Source: three-view drawing plus pictorial views. Frame: mm from the lowest corner of the part. Round coordinates to 2 decimals unless told otherwise and drop trailing zeros. Loops run counter-clockwise (first coordinate to the right, second up) from the corner with the lowest first, then second, coordinate; pieces in that order, holes last. Notation, with made-up numbers: M -18.75,27.5 L 13.25,27.5 A27 cw 13.25,49.5 Z; hole C -37,56.25 d5. An arc over 180 degrees is marked long. Answer as a JSON object with one key per item and string values.
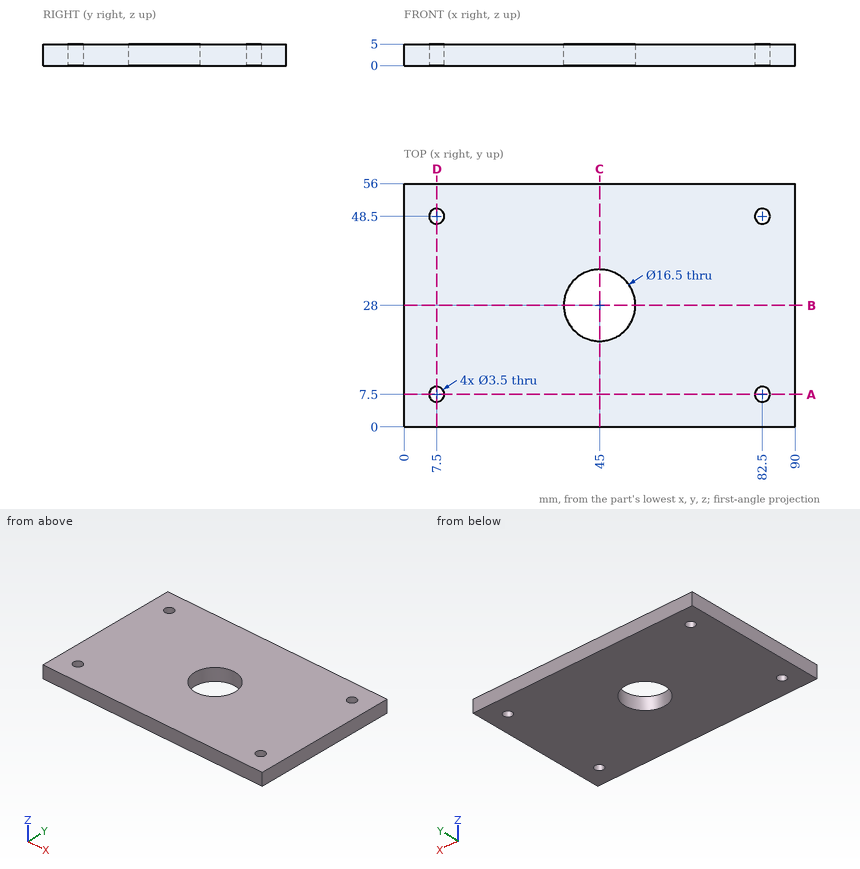
1) Cut plane B-B on y = 28. Return the cut outline in (x, z), and give its area (4 significant figures).
Geometry results:
{"outline": "M 0,0 L 36.75,0 L 36.75,5 L 0,5 Z; M 53.25,0 L 90,0 L 90,5 L 53.25,5 Z", "area": "367.5 mm2"}
2) First-contact query: pin 1 (2 mm diameter, centred on x = 46.5, y = 45, fed in from -Z). Flat tip, straight axial feed; report the tip coordinate or a pass-through.
Geometry results:
{"pin 1": "z = 0"}
3) Cut plane A-A on y = 7.5. Return the cut outline in (x, z).
Geometry results:
{"outline": "M 0,0 L 5.75,0 L 5.75,5 L 0,5 Z; M 9.25,0 L 80.75,0 L 80.75,5 L 9.25,5 Z; M 84.25,0 L 90,0 L 90,5 L 84.25,5 Z"}
4) Line query: probe 1 along Y at (x, z) = (7.5, 1.95); probe 2 along Y at (x, z) = (45, 3.1); probe 3 along X at (y, z) = (28.5, 2.65). Output: solid intervals per line, ascending.
Geometry results:
{"probe 1": "0 to 5.75, 9.25 to 46.75, 50.25 to 56", "probe 2": "0 to 19.75, 36.25 to 56", "probe 3": "0 to 36.77, 53.23 to 90"}
5) Cut plane C-C on x = 45. Return the cut outline in (y, z), and give its area (4 significant figures).
Geometry results:
{"outline": "M 0,0 L 19.75,0 L 19.75,5 L 0,5 Z; M 36.25,0 L 56,0 L 56,5 L 36.25,5 Z", "area": "197.5 mm2"}
6) Cut plane D-D on x = 7.5. Return the cut outline in (y, z), and give its area (3 significant figures).
Geometry results:
{"outline": "M 0,0 L 5.75,0 L 5.75,5 L 0,5 Z; M 9.25,0 L 46.75,0 L 46.75,5 L 9.25,5 Z; M 50.25,0 L 56,0 L 56,5 L 50.25,5 Z", "area": "245 mm2"}
